CAD build for the part. Positions are in the model's coordinates, mm. A direction names the side the tool comes from. Give positions to 0.01 mm unless a question says otherwise; leave off trailing zeros. Write each loop counter-clockwise with the first axis right and the second up, starting at its lowest first coordinate (ties: lowest second). Pieces come first, ordered by that corner, then holes. Notation, with made-up numbers: (-5, 54.5) -> (35, 54.5) arc R13 ccw to (35, 68.5) -> close; hole circle Ø2 at (33, -34.5). An arc over 180 degrees is marked (long way). Answer as a JSON object with one key per item and string values.
```python
from build123d import *

# Parameters (mm, degrees)
SKETCH1_W           = 760
SKETCH1_H           = 350
BOSS_EXTRUDE1_DEPTH = 38
SKETCH2_R           = 65
SKETCH2_R_2         = 55
SKETCH2_R_3         = 45
CUT_EXTRUDE1_DEPTH  = 39
SKETCH4_R           = 75
CUT_EXTRUDE2_DEPTH  = 7
SKETCH5_R           = 70
CUT_EXTRUDE3_DEPTH  = 7
SKETCH12_R          = 3
CUT_EXTRUDE6_DEPTH  = 39
SKETCH15_OUTSIDE_W  = 929.516
SKETCH15_OUTSIDE_H  = 519.516
CUT_EXTRUDE7_DEPTH  = 39
FILLET1_R           = 30
SKETCH16_W          = 760
SKETCH16_H          = 350
CUT_EXTRUDE8_DEPTH  = 18
SKETCH17_R          = 80
SKETCH17_R_2        = 3
CUT_EXTRUDE9_DEPTH  = 7
SKETCH18_R          = 3
CUT_EXTRUDE10_DEPTH = 20


with BuildPart() as part:
    # Sketch1 → Boss-Extrude1 (new body)
    with BuildSketch(Plane.XY):
        with Locations((42.843137255, 32.696078431)):
            Rectangle(SKETCH1_W, SKETCH1_H)
    extrude(amount=BOSS_EXTRUDE1_DEPTH)

    # Sketch2 → Cut-Extrude1 (cut, through all)
    with BuildSketch(Plane.XY.offset(38)):
        with Locations((245.403137255, 24.656078431)):
            Circle(SKETCH2_R)
        with Locations((91.403137255, 24.656078431)):
            Circle(SKETCH2_R_2)
        with Locations((-54.006862745, 24.656078431)):
            Circle(SKETCH2_R_3)
    extrude(amount=-CUT_EXTRUDE1_DEPTH, mode=Mode.SUBTRACT)

    # Sketch4 → Cut-Extrude2 (cut)
    with BuildSketch(Plane.XY.offset(38)):
        with Locations((-54.006862745, 24.656078431)):
            Circle(SKETCH4_R)
    extrude(amount=-CUT_EXTRUDE2_DEPTH, mode=Mode.SUBTRACT)

    # Sketch5 → Cut-Extrude3 (cut)
    with BuildSketch(Plane.XY.offset(38)):
        with Locations((91.403137255, 24.656078431)):
            Circle(SKETCH5_R)
    extrude(amount=-CUT_EXTRUDE3_DEPTH, mode=Mode.SUBTRACT)

    # Sketch12 → Cut-Extrude6 (cut, through all)
    with BuildSketch(Plane.XY.offset(38)):
        with Locations((-54.006862745, 84.656078431)):
            Circle(SKETCH12_R)
        with Locations((-2.045338518, -5.343921569)):
            Circle(SKETCH12_R)
        with Locations((-105.968386972, -5.343921569)):
            Circle(SKETCH12_R)
        with Locations((91.403137255, 84.656078431)):
            Circle(SKETCH12_R)
        with Locations((143.364661482, -5.343921569)):
            Circle(SKETCH12_R)
        with Locations((39.441613028, -5.343921569)):
            Circle(SKETCH12_R)
    extrude(amount=-CUT_EXTRUDE6_DEPTH, mode=Mode.SUBTRACT)

    # Sketch15 outside → Cut-Extrude7 (cut, through all)
    with BuildSketch(Plane.XY.offset(38)):
        with Locations((42.843, 32.696)):
            Rectangle(SKETCH15_OUTSIDE_W, SKETCH15_OUTSIDE_H)
        with BuildLine():
            Line((-277.156862745, 207.696078431), (362.843137255, 207.696078431))
            ThreePointArc((362.843137255, 207.696078431), (405.269544126, 190.122485303), (422.843137255, 147.696078431))
            Line((422.843137255, 147.696078431), (422.843137255, -82.303921569))
            ThreePointArc((422.843137255, -82.303921569), (405.269544126, -124.73032844), (362.843137255, -142.303921569))
            Line((362.843137255, -142.303921569), (-277.156862745, -142.303921569))
            ThreePointArc((-277.156862745, -142.303921569), (-319.583269616, -124.73032844), (-337.156862745, -82.303921569))
            Line((-337.156862745, -82.303921569), (-337.156862745, 147.696078431))
            ThreePointArc((-337.156862745, 147.696078431), (-319.583269616, 190.122485303), (-277.156862745, 207.696078431))
        make_face(mode=Mode.SUBTRACT)
    extrude(amount=-CUT_EXTRUDE7_DEPTH, mode=Mode.SUBTRACT)

    # Fillet1
    fillet1_edges = [part.edges().sort_by_distance(p)[0] for p in [
        (-337.156862745, 32.696078431, 38),
        (42.843137255, -142.303921569, 38),
        (422.843137255, 32.696078431, 38),
        (42.843137255, 207.696078431, 38),
        (405.269544126, -124.73032844, 38),
        (-319.583269616, -124.73032844, 38),
        (-319.583269616, 190.122485303, 38),
        (405.269544126, 190.122485303, 38),
    ]]
    fillet(fillet1_edges, radius=FILLET1_R)

    # Sketch16 → Cut-Extrude8 (cut)
    with BuildSketch(Plane(origin=(0, 0, 0), x_dir=(-1, 0, 0), z_dir=(0, 0, -1))):
        with Locations((-42.843137255, 32.696078431)):
            Rectangle(SKETCH16_W, SKETCH16_H)
    extrude(amount=-CUT_EXTRUDE8_DEPTH, mode=Mode.SUBTRACT)

    # Sketch17 → Cut-Extrude9 (cut)
    with BuildSketch(Plane.XY.offset(38)):
        with Locations((245.403137255, 24.656078431)):
            Circle(SKETCH17_R)
        with Locations((245.403137255, 94.656078431)):
            Circle(SKETCH17_R_2, mode=Mode.SUBTRACT)
        with Locations((306.02491552, -10.343921569)):
            Circle(SKETCH17_R_2, mode=Mode.SUBTRACT)
        with Locations((184.78135899, -10.343921569)):
            Circle(SKETCH17_R_2, mode=Mode.SUBTRACT)
    extrude(amount=-CUT_EXTRUDE9_DEPTH, mode=Mode.SUBTRACT)

    # Sketch18 → Cut-Extrude10 (cut)
    with BuildSketch(Plane.XY.offset(38)):
        with Locations((245.403137255, 94.656078431)):
            Circle(SKETCH18_R)
        with Locations((184.78135899, -10.343921569)):
            Circle(SKETCH18_R)
        with Locations((306.02491552, -10.343921569)):
            Circle(SKETCH18_R)
    extrude(amount=-CUT_EXTRUDE10_DEPTH, mode=Mode.SUBTRACT)


solid = part.part
```
1) Slice it at B-B (y = -65.5). List the corners of the cut face in (x, z).
Model answer:
{"outline": "(-335.44, 18) -> (421.13, 18) arc R30 ccw to (392.84, 38) -> (-307.16, 38) arc R30 ccw to start"}
2) Mould opens along X. For faces 3 (the flat face through (127.4, 66.5, 31)), 4 (the cylindrical face through (-324.688, 34.306, 32.345)), 5 (the cylindrical face through (38.363, -129.835, 32.345)), 6 (the cylindrical face through (321.709, 48.686, 34.549)) say: released by +X, released by -X, zero draft, split by the parting line, or undercut.
Model answer:
{"face 3": "undercut", "face 4": "released by -X", "face 5": "zero draft", "face 6": "undercut"}
3) Slice it at D-D (z = 24.75). State how many separate pieces and enclosed holes the cut face has, then the cut area to 3 significant figures.
Model answer:
{"separate pieces": "1", "enclosed holes": "12", "area": "223,000 mm2"}
4) Pin check, flat tips, straight feed: pin 1 (2 mm diameter, centred on y = 147, z = 35, fed in from -X); pin 2 (1.5 mm diameter, centred on y = 136.5, z = 28, fed in from -X); pin 3 (3.5 mm diameter, centred on x = -54.01, y = 84.66, fed in from +Z); pin 4 (10 mm diameter, centred on y = 169.5, z = 21.5, fed in from -X). Stop position of each tip, or through.
Model answer:
{"pin 1": "stops at x = -322.12", "pin 2": "stops at x = -330.17", "pin 3": "passes through", "pin 4": "stops at x = -332.52"}
5) 3-axis set-ups, long thin cutter, end or side, ignore diameter. For faces 1 (the cylindrical face through (35.854, -17.938, 34.549)), 2 (the cylindrical face through (275.4, -33.01, 24.59)): which of +Z, -Z, +X, -X, +Y, -Y reach the whole face in a straight line?
Model answer:
{"face 1": "+Z", "face 2": "+Z, -Z"}
6) Slice it at C-C (x = -222). List the corners of the cut face in (y, z).
Model answer:
{"outline": "(-140.59, 18) -> (205.98, 18) arc R30 ccw to (177.7, 38) -> (-112.3, 38) arc R30 ccw to start"}
7) Slice it at A-A (x = 128). List the corners of the cut face in (y, z).
Model answer:
{"outline": "(-140.59, 18) -> (-16.4, 18) -> (-16.4, 31) -> (-35.02, 31) -> (-35.02, 38) -> (-112.3, 38) arc R30 ccw to start; (65.71, 18) -> (205.98, 18) arc R30 ccw to (177.7, 38) -> (84.33, 38) -> (84.33, 31) -> (65.71, 31) -> close"}
8) Wall check: probe 1 along X at (y, z) = (26, 23.25); probe 2 along X at (y, z) = (10, 34); probe 3 along Z at (x, y) = (266, -50). Give the ranges that are in metal, low to high.
Model answer:
{"probe 1": "x = -332.99 to -98.99, -9.03 to 36.42, 146.39 to 180.42, 310.39 to 418.68", "probe 2": "x = -322.12 to -127.56, 19.55 to 22.95, 159.85 to 166.76, 324.05 to 407.81", "probe 3": "z = 18 to 31"}
